Geometry: see drawing. Coordinates: mm, zero at the bounding-box minimum. A direction names the side the tool comes from. Coordinates: 2 decimals unless noted, no trailing zeros. Write each loop counter-clockwise with the first axis right and the second up, starting at its lowest first coordinate (ties: lowest second). Pieces come first, ordered by that corner, then holes. Notation, with made-up numbers: M 87.25,11 L 133.25,11 A31 ccw 133.25,42 Z; hole C -26.5,25 d6. An arc over 180 degrees is marked long. Answer as CSV lines item,"result". Start each with the question number.
1. Reachability of the marked faces 4, 5 and 6 from +Z, -Z, +X, -X, +Y, -Y: full face, straight path, thin tool, end or side. Return the list, or none.
2. Line query: probe 1 along X at (y, z) = (11, 50); probe 2 along Y at (x, z) = (165.5, 31.5); probe 3 along Z at (x, y) = (140.5, 12.5). Output: solid intervals per line, ascending. Write a range as [from, to].
3. Mould query, pull axis Y, two halves, no side actions, for the marked faces 1, 2 and 3. Classes: pulls with the +Y half, pulls with the -Y half, needs draft (parallel to the pull), parting line crosses it, or undercut.
4. Contact query for flat-ended pins moving along their axis: pin 1 Ø1 at (y, z) = (64.5, 70.5) entering from -X; pin 2 Ø1 at (y, z) = (21.5, 132) entering from -X; pin 3 Ø22 at (x, y) = (124, 10) entering from +Z. Output: stop coordinate, or through.
5. Section C-C on x = 108.5. Return the cut outline in (y, z).
6. Section A-A on y = 81. Return the cut outline in (x, z), plus the area to 3 significant figures.
7. Section B-B on z = 100. Return the cut outline in (x, y), plus the area to 3 significant figures.
8. Section D-D on z = 172. Return the cut outline in (x, y).
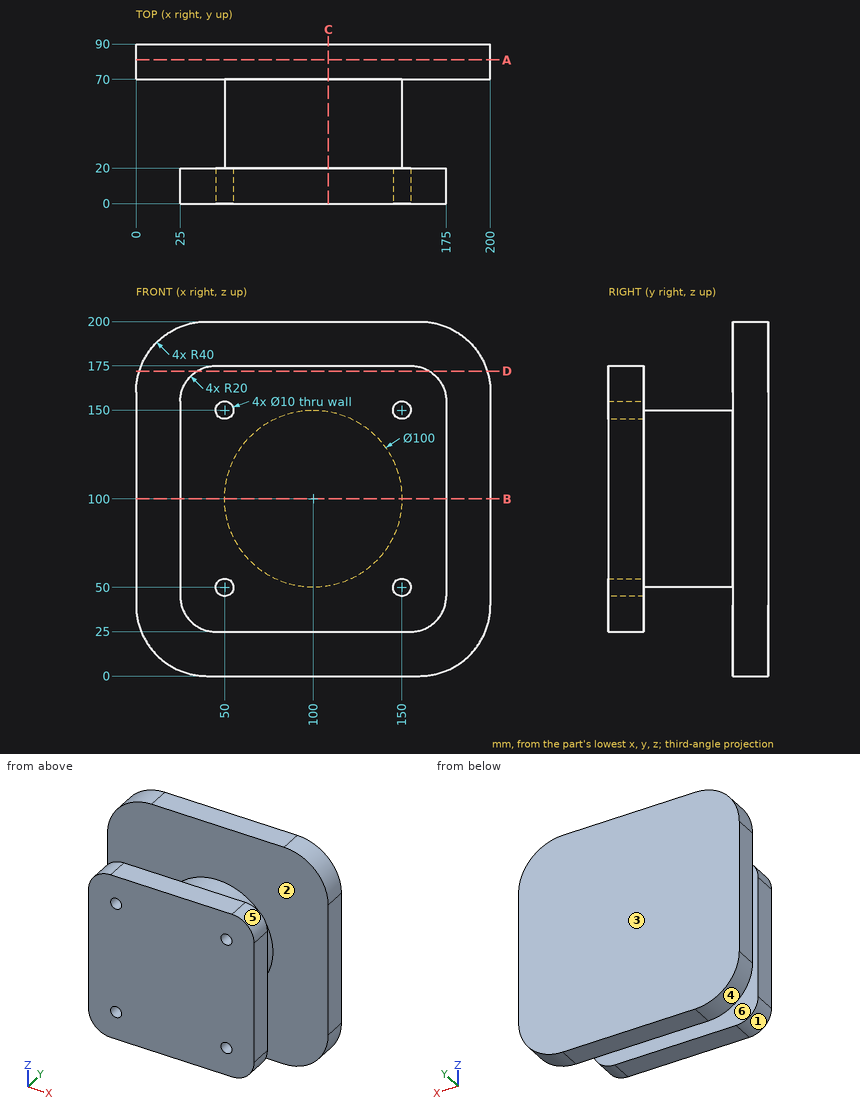
Values:
1,face 4,"-Z, -X, +Y, -Y"
1,face 5,"+Z, +X, -Y"
1,face 6,"none"
2,probe 1,"[25, 45], [55, 145], [155, 175]"
2,probe 2,"[0, 20], [70, 90]"
2,probe 3,"[25, 175]"
3,face 1,"needs draft"
3,face 2,"undercut"
3,face 3,"pulls with the +Y half"
4,pin 1,"x = 59.27"
4,pin 2,"x = 61.17"
4,pin 3,"z = 175"
5,outline,"M 0,25 L 20,25 L 20,50.73 L 70,50.73 L 70,0 L 90,0 L 90,200 L 70,200 L 70,149.27 L 20,149.27 L 20,175 L 0,175 Z"
6,outline,"M 0,40 A40 ccw 40,0 L 160,0 A40 ccw 200,40 L 200,160 A40 ccw 160,200 L 40,200 A40 ccw 0,160 Z"
6,area,"38,600 mm²"
7,outline,"M 0,70 L 50,70 L 50,20 L 25,20 L 25,0 L 175,0 L 175,20 L 150,20 L 150,70 L 200,70 L 200,90 L 0,90 Z"
7,area,"12,000 mm²"
8,outline,"M 1.84,70 L 198.16,70 L 198.16,90 L 1.84,90 Z; M 34.46,0 L 165.54,0 L 165.54,20 L 34.46,20 Z"
